```python
from build123d import *

# Parameters (mm, degrees)
SKETCH1_W           = 373.38
SKETCH1_H           = 309.88
BOSS_EXTRUDE1_DEPTH = 12.7
SKETCH2_W           = 347.98
SKETCH2_H           = 281.94
BOSS_EXTRUDE2_DEPTH = 292.1
SKETCH3_W           = 322.58
SKETCH3_H           = 279.4
CUT_EXTRUDE1_DEPTH  = 266.7
SKETCH4_R           = 6.35
CUT_EXTRUDE2_DEPTH  = 5.08
SKETCH5_W           = 373.38
SKETCH5_H           = 5.08
BOSS_EXTRUDE3_DEPTH = 12.7


with BuildPart() as part:
    # Sketch1 → Boss-Extrude1 (new body)
    with BuildSketch(Plane.XY):
        Rectangle(SKETCH1_W, SKETCH1_H)
    extrude(amount=-BOSS_EXTRUDE1_DEPTH)

    # Sketch2 → Boss-Extrude2 (add)
    with BuildSketch(Plane(origin=(0, 0, -12.7), x_dir=(-1, 0, 0), z_dir=(0, 0, -1))):
        with Locations((0, 1.27)):
            Rectangle(SKETCH2_W, SKETCH2_H)
    extrude(amount=BOSS_EXTRUDE2_DEPTH)

    # Sketch3 → Cut-Extrude1 (cut)
    with BuildSketch(Plane(origin=(0, 142.24, 0), x_dir=(1, 0, 0), z_dir=(0, 1, 0))):
        with Locations((0, 152.4)):
            Rectangle(SKETCH3_W, SKETCH3_H)
    extrude(amount=-CUT_EXTRUDE1_DEPTH, mode=Mode.SUBTRACT)

    # Sketch4 → Cut-Extrude2 (cut)
    with BuildSketch(Plane.XY):
        with Locations((-38.1, 0)):
            Circle(SKETCH4_R)
        with Locations((38.1, 0)):
            Circle(SKETCH4_R)
    extrude(amount=-CUT_EXTRUDE2_DEPTH, mode=Mode.SUBTRACT)

    # Sketch5 → Boss-Extrude3 (add)
    with BuildSketch(Plane.XY):
        with Locations((0, 157.48)):
            Rectangle(SKETCH5_W, SKETCH5_H)
    extrude(amount=-BOSS_EXTRUDE3_DEPTH)


solid = part.part
```
Check sheet for the modelled part. Datum: model origin and axes. Units: mm. A direction names the side the tool comes from. Give positions to 0.01 mm unless a question says otherwise; leave off trailing zeros. Order: outer loops, then holes, each group sorted by start corner. A loop starts at its lowest first (then second) coordinate and runs counter-clockwise, first axis right, second up. Notation, with made-up numbers: M 30,-30.5 L 39,-30.5 A20 cw 39,-18.5 Z; hole C 37,-13.75 d3. An arc over 180 degrees is marked long. Answer in a Markdown table with one row per item. Add a question column.
Q1. Sectioned sample at C-C, the plane z = -54.5. Record the boundary of the cut face in (x, y), and give its area (3 significant figures).
Q2. Sectioned sample at A-A, the plane x = 129. Record the boundary of the cut face in (y, z).
Q3. Access from +Z, -Z, +X, -X, +Y, -Y to the whole of each face (thin tool, end or side, straight path). Record for faces 4 (the flat face through (-161.29, 11, -150)), 5 (the flat face through (-173.99, -1, -157)), 6 (the flat face through (2, -139.7, -157)), 7 (the flat face through (1, 142.24, -299)).
Q4. Gauge pin test, flat ends, axial feed: pin 1 Ø1.5 at (x, z) = (52, -62) entering from +Y; pin 2 Ø3 at (y, z) = (-111, -143) entering from +X; pin 3 Ø10 at (x, y) = (-36, -2) entering from +Z; pin 4 Ø3 at (x, z) = (-61, -74.5) entering from -Y. Record the tip position at first contact, or that the pin passes through.
Q5. Thickness scan on L1, parallel to Z at x = -27.5, y = 130; L2, parallel to X at y = 120, z = -265.5; L3, parallel to Y at x = 38.1, z = -2.85. Record the ranges inside material, lowest first.
Q6. Sectioned sample at D-D, the plane y = -133. Record the boundary of the cut face in (x, z).
Q7. Sectioned sample at B-B, the plane y = 97. Record the boundary of the cut face in (x, z).
Q8. Release check for a two-part mould opening along Y. For faces 1 (the cylindrical face through (-32.043, 1.907, -2.504)), 2 (the flat face through (-3, 160.02, -6)), 3 (the flat face through (-3, -154.94, -6)) record: released by +Y, released by -Y, zero draft, split by the parting line, or undercut.
Verdict:
| question | item | result |
|---|---|---|
| 1 | outline | M -173.99,-139.7 L 173.99,-139.7 L 173.99,142.24 L 161.29,142.24 L 161.29,-124.46 L -161.29,-124.46 L -161.29,142.24 L -173.99,142.24 Z |
| 1 | area | 12,100 mm² |
| 2 | outline | M -154.94,-12.7 L -139.7,-12.7 L -139.7,-304.8 L 142.24,-304.8 L 142.24,-292.1 L -124.46,-292.1 L -124.46,-12.7 L 160.02,-12.7 L 160.02,0 L -154.94,0 Z |
| 3 | face 4 | +Y |
| 3 | face 5 | -Z, -X, +Y, -Y |
| 3 | face 6 | -Z, +X, -X, -Y |
| 3 | face 7 | -Z, +X, -X, +Y |
| 4 | pin 1 | y = -124.46 |
| 4 | pin 2 | x = 173.99 |
| 4 | pin 3 | z = 0 |
| 4 | pin 4 | y = -139.7 |
| 5 | L1 | -304.8 to -292.1, -12.7 to 0 |
| 5 | L2 | -173.99 to -161.29, 161.29 to 173.99 |
| 5 | L3 | -154.94 to -6.35, 6.35 to 160.02 |
| 6 | outline | M -186.69,-12.7 L -173.99,-12.7 L -173.99,-304.8 L 173.99,-304.8 L 173.99,-12.7 L 186.69,-12.7 L 186.69,0 L -186.69,0 Z |
| 7 | outline | M -186.69,-12.7 L -173.99,-12.7 L -173.99,-304.8 L 173.99,-304.8 L 173.99,-12.7 L 186.69,-12.7 L 186.69,0 L -186.69,0 Z; hole M -161.29,-292.1 L 161.29,-292.1 L 161.29,-12.7 L -161.29,-12.7 Z |
| 8 | face 1 | undercut |
| 8 | face 2 | released by +Y |
| 8 | face 3 | released by -Y |
